Input: dimensioned drawing with shaded views. Units: mm. Origin: part minimum x, y, z. A direction names the side the tool comes from. Round coordinates to 2 decimals unless told otherwise and drop trailing zeros. Loops run counter-clockwise (first coordinate to the right, second up) from the corner with the lowest first, then second, coordinate; pieces in that order, holes last. Notation, with made-up numbers: (-16, -17) - (6, -17) arc R10 cw to (6, 1) - close; hole circle Ø6 at (84, 4). An arc over 180 degrees is marked (long way). One line per question, with ' | ' between items.
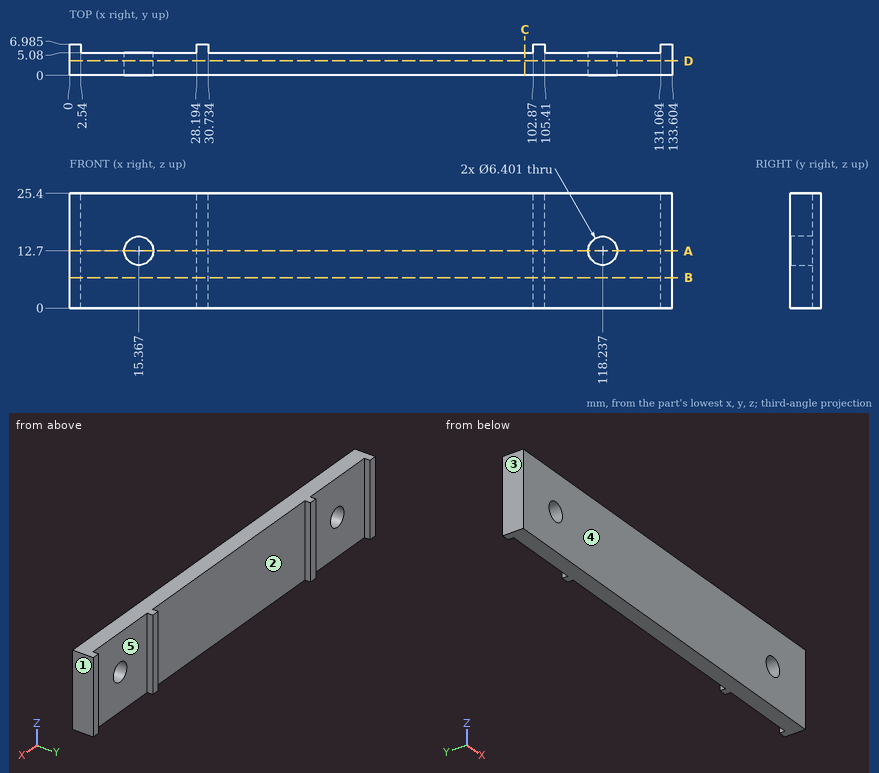
1. Access query for the marked faces 1 and 2. Directions: +Z, -Z, +X, -X, +Y, -Y. A direction counts if a zero-diameter tool reaches every point of the face in a straight line with its end or side. Return the directions, or none.
Worked out:
face 1: +Z, -Z, +X, +Y, -Y | face 2: +Z, -Z, +Y
2. Contact query for a flat-ended pin moving along its axis: P1, Ø12.5, axis at x = 12.5, z = 9, coming from the +Y side. Output: stop coordinate, or through.
Worked out:
P1: stops at y = 5.08
3. Section query C-C, the plane x = 101. Return loops of the section in (y, z).
Worked out:
outline: (0, 0) - (5.08, 0) - (5.08, 25.4) - (0, 25.4) - close
4. Section query B-B, the plane z = 6.75. Return loops of the section in (x, y) (3 decimals).
Worked out:
outline: (0, 0) - (133.604, 0) - (133.604, 6.985) - (131.064, 6.985) - (131.064, 5.08) - (105.41, 5.08) - (105.41, 6.985) - (102.87, 6.985) - (102.87, 5.08) - (30.734, 5.08) - (30.734, 6.985) - (28.194, 6.985) - (28.194, 5.08) - (2.54, 5.08) - (2.54, 6.985) - (0, 6.985) - close
5. Material intervals for probe 1 along X at (y, z) = (2.75, 12.5); probe 2 along X at (y, z) = (5.75, 18); probe 3 along X at (y, z) = (2.5, 14.25), sorted ascending.
Worked out:
probe 1: x = 0 to 12.17, 18.56 to 115.04, 121.43 to 133.6 | probe 2: x = 0 to 2.54, 28.19 to 30.73, 102.87 to 105.41, 131.06 to 133.6 | probe 3: x = 0 to 12.57, 18.17 to 115.44, 121.04 to 133.6
6. Section query D-D, the plane y = 3.25. Return loops of the section in (x, z).
Worked out:
outline: (0, 0) - (133.6, 0) - (133.6, 25.4) - (0, 25.4) - close; hole circle Ø6.4 at (15.37, 12.7); hole circle Ø6.4 at (118.24, 12.7)
7. Section query A-A, the plane z = 12.7. Return loops of the section in (x, y) (1 decimal).
Worked out:
outline: (0, 0) - (12.2, 0) - (12.2, 5.1) - (2.5, 5.1) - (2.5, 7) - (0, 7) - close; (18.6, 0) - (115, 0) - (115, 5.1) - (105.4, 5.1) - (105.4, 7) - (102.9, 7) - (102.9, 5.1) - (30.7, 5.1) - (30.7, 7) - (28.2, 7) - (28.2, 5.1) - (18.6, 5.1) - close; (121.4, 0) - (133.6, 0) - (133.6, 7) - (131.1, 7) - (131.1, 5.1) - (121.4, 5.1) - close
8. Mould query, pull axis X, two halves, no side actions, for the marked faces 3, 4 and 5. Classes: released by +X, released by -X, zero draft, split by the parting line, or undercut.
Worked out:
face 3: released by -X | face 4: zero draft | face 5: undercut
